```python
from build123d import *

# Parameters (mm, degrees)
SKETCH1_W           = 17
SKETCH1_H           = 17
BOSS_EXTRUDE1_DEPTH = 2
SKETCH2_W           = 15.2
SKETCH2_H           = 15.2
CUT_EXTRUDE1_DEPTH  = 1.6
SKETCH3_W           = 1.125
SKETCH3_H           = 1.125
CUT_EXTRUDE2_DEPTH  = 3


with BuildPart() as part:
    # Sketch1 → Boss-Extrude1 (new body)
    with BuildSketch(Plane(origin=(0, 0, 0), x_dir=(1, 0, 0), z_dir=(0, 1, 0))):
        Rectangle(SKETCH1_W, SKETCH1_H)
    extrude(amount=BOSS_EXTRUDE1_DEPTH)

    # Sketch2 → Cut-Extrude1 (cut)
    with BuildSketch(Plane.XZ):
        Rectangle(SKETCH2_W, SKETCH2_H)
    extrude(amount=-CUT_EXTRUDE1_DEPTH, mode=Mode.SUBTRACT)

    # Sketch3 → Cut-Extrude2 (cut, through all)
    with BuildSketch(Plane(origin=(0, 2, 0), x_dir=(1, 0, 0), z_dir=(0, 1, 0))):
        with Locations((-4.0625, 5.6875)):
            Rectangle(SKETCH3_W, SKETCH3_H)
        with Locations((-2.4375, 5.6875)):
            Rectangle(SKETCH3_W, SKETCH3_H)
        with Locations((2.4375, 5.6875)):
            Rectangle(SKETCH3_W, SKETCH3_H)
        with Locations((4.0625, 5.6875)):
            Rectangle(SKETCH3_W, SKETCH3_H)
        with Locations((5.6875, 4.0625)):
            Rectangle(SKETCH3_W, SKETCH3_H)
        with Locations((5.6875, 2.4375)):
            Rectangle(SKETCH3_W, SKETCH3_H)
        with Locations((5.6875, 0.8125)):
            Rectangle(SKETCH3_W, SKETCH3_H)
        with Locations((-5.6875, 4.0625)):
            Rectangle(SKETCH3_W, SKETCH3_H)
        with Locations((-5.6875, 2.4375)):
            Rectangle(SKETCH3_W, SKETCH3_H)
        with Locations((-5.6875, 0.8125)):
            Rectangle(SKETCH3_W, SKETCH3_H)
        with Locations((-4.0625, -0.8125)):
            Rectangle(SKETCH3_W, SKETCH3_H)
        with Locations((-2.4375, -2.4375)):
            Rectangle(SKETCH3_W, SKETCH3_H)
        with Locations((-0.8125, -4.0625)):
            Rectangle(SKETCH3_W, SKETCH3_H)
        with Locations((0.8125, -4.0625)):
            Rectangle(SKETCH3_W, SKETCH3_H)
        with Locations((2.4375, -2.4375)):
            Rectangle(SKETCH3_W, SKETCH3_H)
        with Locations((4.0625, -0.8125)):
            Rectangle(SKETCH3_W, SKETCH3_H)
        with Locations((-0.8125, 4.0625)):
            Rectangle(SKETCH3_W, SKETCH3_H)
        with Locations((0.8125, 4.0625)):
            Rectangle(SKETCH3_W, SKETCH3_H)
        with Locations((-4.0625, 4.0625)):
            Rectangle(SKETCH3_W, SKETCH3_H)
        with Locations((-4.0625, 2.4375)):
            Rectangle(SKETCH3_W, SKETCH3_H)
        with Locations((-2.4375, 0.8125)):
            Rectangle(SKETCH3_W, SKETCH3_H)
        with Locations((-2.4375, 2.4375)):
            Rectangle(SKETCH3_W, SKETCH3_H)
        with Locations((-2.4375, 4.0625)):
            Rectangle(SKETCH3_W, SKETCH3_H)
        with Locations((-0.8125, 2.4375)):
            Rectangle(SKETCH3_W, SKETCH3_H)
        with Locations((0.8125, 2.4375)):
            Rectangle(SKETCH3_W, SKETCH3_H)
        with Locations((2.4375, 0.8125)):
            Rectangle(SKETCH3_W, SKETCH3_H)
        with Locations((2.4375, 2.4375)):
            Rectangle(SKETCH3_W, SKETCH3_H)
        with Locations((2.4375, 4.0625)):
            Rectangle(SKETCH3_W, SKETCH3_H)
        with Locations((4.0625, 2.4375)):
            Rectangle(SKETCH3_W, SKETCH3_H)
        with Locations((4.0625, 0.8125)):
            Rectangle(SKETCH3_W, SKETCH3_H)
        with Locations((2.4375, -0.8125)):
            Rectangle(SKETCH3_W, SKETCH3_H)
        with Locations((0.8125, -0.8125)):
            Rectangle(SKETCH3_W, SKETCH3_H)
        with Locations((-2.4375, -0.8125)):
            Rectangle(SKETCH3_W, SKETCH3_H)
        with Locations((-0.8125, -2.4375)):
            Rectangle(SKETCH3_W, SKETCH3_H)
        with Locations((0.8125, -2.4375)):
            Rectangle(SKETCH3_W, SKETCH3_H)
        with Locations((-0.8125, -0.8125)):
            Rectangle(SKETCH3_W, SKETCH3_H)
        with Locations((-4.0625, 0.8125)):
            Rectangle(SKETCH3_W, SKETCH3_H)
        with Locations((-0.8125, 0.8125)):
            Rectangle(SKETCH3_W, SKETCH3_H)
        with Locations((0.8125, 0.8125)):
            Rectangle(SKETCH3_W, SKETCH3_H)
        with Locations((4.0625, 4.0625)):
            Rectangle(SKETCH3_W, SKETCH3_H)
        with Locations((5.6875, -0.8125)):
            Rectangle(SKETCH3_W, SKETCH3_H)
        with Locations((4.0625, -2.4375)):
            Rectangle(SKETCH3_W, SKETCH3_H)
        with Locations((2.4375, -4.0625)):
            Rectangle(SKETCH3_W, SKETCH3_H)
        with Locations((0.8125, -5.6875)):
            Rectangle(SKETCH3_W, SKETCH3_H)
        with Locations((-0.8125, -5.6875)):
            Rectangle(SKETCH3_W, SKETCH3_H)
        with Locations((-2.4375, -4.0625)):
            Rectangle(SKETCH3_W, SKETCH3_H)
        with Locations((-4.0625, -2.4375)):
            Rectangle(SKETCH3_W, SKETCH3_H)
        with Locations((-5.6875, -0.8125)):
            Rectangle(SKETCH3_W, SKETCH3_H)
    extrude(amount=-CUT_EXTRUDE2_DEPTH, mode=Mode.SUBTRACT)


solid = part.part
```
CAD build for the part. Positions are in the model's coordinates, mm. A direction names the side the tool comes from. Round coordinates to 2 decimals unless told otherwise and drop trailing zeros. Order: outer loops, then holes, each group sorted by start corner. A loop starts at its lowest first (then second) coordinate and runs counter-clockwise, first axis right, second up.
Q1. Which spindle directions (+Z, -Z, +X, -X, +Y, -Y) get a long thin tool onto all of the face, cutting with end or side? Do faces 4 (the flat face through (0, 1, 7.6)), 5 (the flat face through (-1, 0, 8)). Say none if no direction does.
Q2. Slice it at B-B (x = -4). State how many separate pieces and enclosed holes the cut face has, and give its area (3 significant figures).
Q3. Two-plate mould, pull along X, no slides. Class faces 1 (the flat face through (8.5, 1, 0)), 2 (the flat face through (7.6, 1, 0)), 3 (the flat face through (0, 1, 8.5)): pulls with the +X half, pulls with the -X half, needs draft (parallel to the pull), parting line crosses it, or undercut.
Q4. Slice it at D-D (x = -5.75). Write the cut outline in (y, z) (3 decimals), and give its area (3 significant figures).
Q5. Slice it at A-A (y = 1.15). Write the cut outline in (x, z), and give its area (3 significant figures).
Q6. Slice it at C-C (z = 3.25). Write the cut outline in (x, y).
Q7. Wall check: L1, parallel to Z at x = 1.5, y = 0.4; L2, parallel to Y at x = -5.25, z = 2. Give the ranges that are in metal, low to high.
Results below:
1. face 4: -Y
1. face 5: +Z, -Z, +X, -X, -Y
2. separate pieces: 7
2. enclosed holes: 0
2. area: 6.98 mm2
3. face 1: pulls with the +X half
3. face 2: undercut
3. face 3: needs draft
4. outline: (0, -8.5) - (2, -8.5) - (2, -4.625) - (1.6, -4.625) - (1.6, -7.6) - (0, -7.6) - close; (0, 7.6) - (1.6, 7.6) - (1.6, 1.375) - (2, 1.375) - (2, 8.5) - (0, 8.5) - close; (1.6, -3.5) - (2, -3.5) - (2, -3) - (1.6, -3) - close; (1.6, -1.875) - (2, -1.875) - (2, -1.375) - (1.6, -1.375) - close; (1.6, -0.25) - (2, -0.25) - (2, 0.25) - (1.6, 0.25) - close
4. area: 7.88 mm2
5. outline: (-8.5, -8.5) - (8.5, -8.5) - (8.5, 8.5) - (-8.5, 8.5) - close; hole (-7.6, -7.6) - (7.6, -7.6) - (7.6, 7.6) - (-7.6, 7.6) - close
5. area: 58.0 mm2
6. outline: (-8.5, 0) - (-7.6, 0) - (-7.6, 1.6) - (7.6, 1.6) - (7.6, 0) - (8.5, 0) - (8.5, 2) - (-8.5, 2) - close
7. L1: z = -8.5 to -7.6, 7.6 to 8.5
7. L2: y = 1.6 to 2
